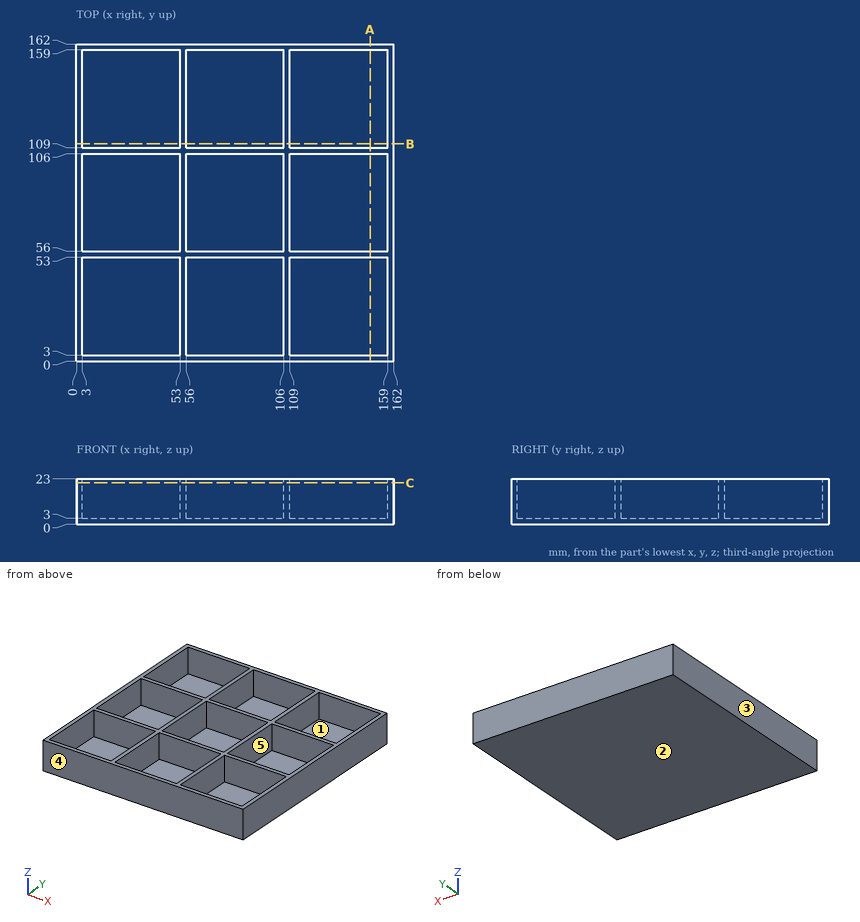
Source: three-view drawing plus pictorial views. Frame: mm from the lowest corner of the part. A direction names the side the tool comes from. Give positions to 0.01 mm unless a question says otherwise; leave off trailing zeros. Order: outer loops, then holes, each group sorted by start corner. A loop starts at its lowest first (then second) coordinate and runs counter-clockwise, first axis right, second up. Notation, with made-up numbers: M 48.25,49.5 L 106.25,49.5 A25 ccw 106.25,82.5 Z; hole C -8.5,-1 d4. An arc over 180 degrees is marked long. Return JSON: item names as keys, results as strings.
1) Section query A-A on x = 150. Output: boundary loops of the cut face in (y, z), and give its area (3 significant figures).
Taken from the geometry:
{"outline": "M 0,0 L 162,0 L 162,23 L 159,23 L 159,3 L 109,3 L 109,23 L 106,23 L 106,3 L 56,3 L 56,23 L 53,23 L 53,3 L 3,3 L 3,23 L 0,23 Z", "area": "726 mm2"}
2) Section query C-C on z = 21. Count the separate pieces of the cut face and the enclosed holes in it, and give its area (3 significant figures).
Taken from the geometry:
{"separate pieces": "1", "enclosed holes": "9", "area": "3,740 mm2"}
3) Mould query, pull axis X, two halves, no side actions, for the marked faces 1, 2 and 3. Classes: released by +X, released by -X, zero draft, split by the parting line, or undercut.
Taken from the geometry:
{"face 1": "undercut", "face 2": "zero draft", "face 3": "released by -X"}
4) Contact query for a flat-ended pin moving along its axis: pin 1 (15 mm diameter, centred on x = 19, y = 91, fed in from +Z). Output: stop coordinate, or through.
Taken from the geometry:
{"pin 1": "stops at z = 3"}
5) Access query for the marked faces 4 and 5. Directions: +Z, -Z, +X, -X, +Y, -Y. A direction counts if a zero-diameter tool reaches every point of the face in a straight line with its end or side. Return the directions, or none.
Taken from the geometry:
{"face 4": "+Z, -Z, +X, -X, -Y", "face 5": "+Z"}
6) Line query: L1, parallel to X at y = 102.5, z = 8; L2, parallel to Z at x = 24, y = 70. Output: solid intervals per line, ascending. Write a range as [from, to].
Taken from the geometry:
{"L1": "x = [0, 3], [53, 56], [106, 109], [159, 162]", "L2": "z = [0, 3]"}
